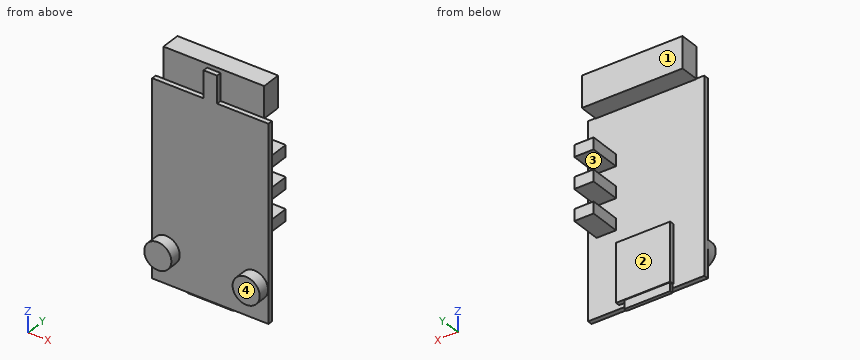
Autodesk Inventor part; units mm, degrees
ref_plane "YZ Plane" through (0, 0, 0) normal (1, 0, 0) x (0, 1, 0)
ref_plane "XZ Plane" through (0, 0, 0) normal (0, 1, 0) x (-1, 0, 0)
ref_plane "XY Plane" through (0, 0, 0) normal (0, 0, 1) x (1, 0, 0)
sketch "Sketch1" plane through (0, 0, 0) normal (0, 1, 0) x (-1, 0, 0)
  line L0 (22.7568, 36.7979) -> (-7.2432, 36.7979)
  line L1 (-7.2432, 36.7979) -> (-7.2432, -13.2021)
  line L2 (-7.2432, -13.2021) -> (22.7568, -13.2021)
  line L3 (22.7568, -13.2021) -> (22.7568, 36.7979)
  line L4 (7.7568, 36.7979) -> (7.7568, 43.7979)
  line L5 (7.7568, 43.7979) -> (9.5068, 43.7979)
  line L6 (9.5068, 43.7979) -> (9.5068, 36.7979)
  line L7 (9.5068, 43.7979) -> (6.0068, 43.7979)
  line L8 (6.0068, 43.7979) -> (6.0068, 36.7979)
  point P0 (0, 0)
  dimension "d0" = 30
  dimension "d1" = 50
  dimension "d2" = 7
  dimension "d3" = 1.75
  dimension "d4" = 3.5
extrude "Extrusion1" add sketch "Sketch1" along normal blind 1.25
sketch "Sketch2" plane through (0, 1.25, 0) normal (0, 1, 0) x (1, 0, 0)
  line L0 (-20.7568, -36.6979) -> (5.2432, -36.6979)
  line L1 (5.2432, -36.6979) -> (5.2432, -44.7979)
  line L2 (5.2432, -44.7979) -> (-20.7568, -44.7979)
  line L3 (-20.7568, -44.7979) -> (-20.7568, -36.6979)
  line L4 (-9.5068, -43.7979) -> (-6.0068, -43.7979)
  line L5 (-6.0068, -43.7979) -> (-9.5068, -43.7979)
  line L6 (-22.7568, 13.2021) -> (-22.7568, -36.7979)
  line L7 (7.2432, -36.7979) -> (7.2432, 13.2021)
  point P0 (0, 0)
  point P1 (-7.7568, -43.7979)
  point P2 (5.2432, -40.7479)
  dimension "d7" = 1
  dimension "d8" = 8.1
  dimension "d9" = 2
  dimension "d10" = 2
extrude "Extrusion2" add sketch "Sketch2" along normal blind 5
sketch "Sketch3" plane through (0, 1.25, 0) normal (0, 1, 0) x (1, 0, 0)
  line L0 (0.0432, -9.7979) -> (5.0432, -9.7979)
  line L1 (5.0432, -9.7979) -> (5.0432, -6.7979)
  line L2 (5.0432, -6.7979) -> (0.0432, -6.7979)
  line L3 (0.0432, -6.7979) -> (0.0432, -9.7979)
  line L4 (0.0432, -17.7979) -> (5.0432, -17.7979)
  line L5 (5.0432, -17.7979) -> (5.0432, -14.7979)
  line L6 (5.0432, -14.7979) -> (0.0432, -14.7979)
  line L7 (0.0432, -14.7979) -> (0.0432, -17.7979)
  line L8 (0.0432, -25.7979) -> (5.0432, -25.7979)
  line L9 (5.0432, -25.7979) -> (5.0432, -22.7979)
  line L10 (5.0432, -22.7979) -> (0.0432, -22.7979)
  line L11 (0.0432, -22.7979) -> (0.0432, -25.7979)
  line L12 (7.2432, -36.7979) -> (7.2432, 13.2021)
  line L13 (7.2432, 13.2021) -> (-22.7568, 13.2021)
  point P0 (0, 0)
  point P1 (-0.1282, -6.8631)
  point P2 (-0.0024, -12.7771)
  point P3 (5.0432, -8.2979)
  point P4 (5.0432, -16.2979)
  point P5 (5.0432, -24.2979)
  point P6 (2.5432, -17.7979)
  point P7 (2.5432, -22.7979)
  dimension "d13" = 5
  dimension "d14" = 3
  dimension "d15" = 5
  dimension "d16" = 3
  dimension "d17" = 5
  dimension "d18" = 3
  dimension "d19" = 2.2
  dimension "d20" = 2.2
  dimension "d21" = 2.2
  dimension "d22" = 20
  dimension "d23" = 5
  dimension "d24" = 5
extrude "Extrusion3" add sketch "Sketch3" along normal blind 8
sketch "Sketch4" plane through (0, 1.25, 0) normal (0, 1, 0) x (1, 0, 0)
  line L0 (-14.7568, -2.7979) -> (-0.7568, -2.7979)
  line L1 (-0.7568, -2.7979) -> (-0.7568, 12.2021)
  line L2 (-0.7568, 12.2021) -> (-14.7568, 12.2021)
  line L3 (-14.7568, 12.2021) -> (-14.7568, -2.7979)
  line L4 (-22.7568, 13.2021) -> (-22.7568, -36.7979)
  line L5 (7.2432, -36.7979) -> (7.2432, 13.2021)
  line L6 (7.2432, 13.2021) -> (-22.7568, 13.2021)
  point P0 (0, 0)
  dimension "d27" = 8
  dimension "d28" = 8
  dimension "d29" = 1
  dimension "d30" = 15
extrude "Extrusion4" add sketch "Sketch4" along normal blind 1.1
sketch "Sketch5" plane through (-0.7568, 1.25, -12.2021) normal (0, 0, -1) x (-1, 0, 0)
  line L0 (2, 0.9) -> (13.8, 0.9)
  line L1 (13.8, 0.9) -> (13.8, 0.017)
  line L2 (13.8, 0.017) -> (2, 0.017)
  line L3 (2, 0.017) -> (2, 0.9)
  line L4 (0, 0) -> (0, 1.1)
  line L5 (14, 0) -> (14, 1.1)
  line L6 (0, 1.1) -> (14, 1.1)
  line L7 (-8, 0) -> (22, 0)
  point P0 (-0.7568, -1.25)
  point P1 (0, 0.55)
  point P2 (2, 0.4585)
  point P3 (14, 0.55)
  point P4 (13.8, 0.4585)
  dimension "d33" = 2
  dimension "d34" = 0.2
  dimension "d35" = 0.2
  dimension "d36" = 0.017
extrude "Extrusion5" add sketch "Sketch5" along normal blind 2.2 contours L0 L1 L2 L3
sketch "Sketch6" plane through (0, 0, 0) normal (0, -1, 0) x (1, 0, 0)
  circle A0 centre (3.6432, -4.7021) radius 3.5
  circle A1 centre (-19.1568, -4.7021) radius 3.5
  line L0 (7.2432, -13.2021) -> (-22.7568, -13.2021)
  line L1 (-22.7568, -13.2021) -> (-22.7568, 36.7979)
  line L2 (7.2432, 36.7979) -> (7.2432, -13.2021)
  point P0 (0, 0)
  dimension "d39" = 7
  dimension "d40" = 7
  dimension "d41" = 8.5
  dimension "d42" = 8.5
  dimension "d43" = 3.6
  dimension "d44" = 3.6
extrude "Extrusion6" add sketch "Sketch6" along normal blind 3
properties part number "Sd card reader"
Input: part model. Units: mm. Frame: model coordinates. Face numbers are marked on the shaded views. A direction names the side the tool comes from. Give positions to 0.01 mm unless a question says otherwise; leave off trailing zeros. Order: outer loops, then holes, each group sorted by start corner. A loop starts at its lowest first (then second) coordinate and runs counter-clockwise, first axis right, second up.
1. Line query: probe 1 along Z at (x, y) = (0.5, 4.75); probe 2 along Z at (x, y) = (1.25, 8.5); probe 3 along Z at (x, y) = (-6, 2.25). Output: solid intervals per line, ascending.
Computed:
probe 1: z = 6.8 to 9.8, 14.8 to 17.8, 22.8 to 25.8, 36.7 to 44.8
probe 2: z = 6.8 to 9.8, 14.8 to 17.8, 22.8 to 25.8
probe 3: z = -12.2 to 2.8, 36.7 to 44.8
2. Set-up query: the marked faces 1, 2, 3 and 4. Return all of +Z, -Z, +X, -X, +Y, -Y with unobstructed straight access to the full face (end or side cutting, diameter ignored); none if empty.
Computed:
face 1: +Z, +X, -X, +Y
face 2: -Z, +X, -X, +Y
face 3: +X, -X, +Y
face 4: +Z, -Z, +X, -X, -Y
3. Cut plane C-C (y = 3.75). Return loops of the section in (x, z).
Computed:
outline: (-20.76, 36.7) - (5.24, 36.7) - (5.24, 44.8) - (-20.76, 44.8) - close; (0.04, 6.8) - (5.04, 6.8) - (5.04, 9.8) - (0.04, 9.8) - close; (0.04, 14.8) - (5.04, 14.8) - (5.04, 17.8) - (0.04, 17.8) - close; (0.04, 22.8) - (5.04, 22.8) - (5.04, 25.8) - (0.04, 25.8) - close
4. Cut plane A-A (y = 8.25). Return loops of the section in (x, z).
Computed:
outline: (0.04, 6.8) - (5.04, 6.8) - (5.04, 9.8) - (0.04, 9.8) - close; (0.04, 14.8) - (5.04, 14.8) - (5.04, 17.8) - (0.04, 17.8) - close; (0.04, 22.8) - (5.04, 22.8) - (5.04, 25.8) - (0.04, 25.8) - close
5. Pin query (flat end, axial travel): pin 1 Ø2.5 at (y, z) = (4, 17) entering from +X; pin 2 Ø11 at (x, z) = (-10.5, -7.5) entering from +Y; pin 3 Ø2.5 at (x, z) = (-10.5, -13) entering from -Y. Return the tip coordinate at first contact, or that it passes through.
Computed:
pin 1: stops at x = 5.04
pin 2: stops at y = 2.35
pin 3: stops at y = 0
6. Cut plane B-B (z = -9.5). Return loops of the section in (x, y).
Computed:
outline: (-22.76, 0) - (7.24, 0) - (7.24, 1.25) - (-0.76, 1.25) - (-0.76, 2.35) - (-14.76, 2.35) - (-14.76, 1.25) - (-22.76, 1.25) - close
